CAD build for the part. Positions are in the model's coordinates, mm. Face numbers are marked on the shaded views. A direction names the side the tool comes from. Round coordinates to 2 decimals unless told otherwise and drop trailing zeros. Loops run counter-clockwise (first coordinate to the right, second up) from the corner with the lowest first, then second, coordinate; pieces in that order, holes last. Notation, with made-up numbers: M 59.5,-27.5 L 79.5,-27.5 A15 ccw 79.5,-17.5 Z; hole C 63.25,-11 d1. An arc over 180 degrees is marked long. Use a Markdown table: item, result. Add a question column.
(1) Two-plate mould, pull along Y, no slides. Class the marked faces 1, 2, 3 and 4: released by +Y, released by -Y, zero draft, split by the parting line, or undercut.
(2) Which spindle directions (+Z, -Z, +X, -X, +Y, -Y) get a long thin tool onto all of the face, cutting with end or side? Do the marked faces 5 and 6. Say none if no direction does.
(3) Band-saw the part on A-A, the plane y = 0. Write the cut outline in (x, z), and give its area (3 significant figures).
(4) Wall check: L1, parallel to Y at x = 0, z = 57; L2, parallel to Y at x = 0, z = 48.5; L3, parallel to Z at x = 21, y = 32. Give the ranges that are in metal, low to high.
(5) Band-saw the part on C-C, the plane z = -35.5. Write the cut outline in (x, y), and give its area (3 significant figures).
(6) Flat gauge pins, fed straight in: P1, Ø10, axis at x = 26, z = 6.5, coming from the -Y side; P2, Ø12, axis at y = 32, z = 14.5, coming from the +X side; P3, Ø1.5, axis at x = -9.5, z = -12.5, coming from the +Y side. Where does each tip first touch, or does it go through?
(7) Band-saw the part on D-D, the plane z = -20. Write the cut outline in (x, y).
from build123d import *

# Parameters (mm, degrees)
F2_R     = 19.05
F3_DEPTH = 6.35
F4_R     = 19.05
F5_DEPTH = 16.002


with BuildPart() as f1:
    # F0 (on Front) → F1 (revolve)
    with BuildSketch(Plane.XZ):
        with BuildLine():
            Line((0, -53.330265), (0, 60.969735))
            Line((0, 60.969735), (-40.845792, 60.969735))
            ThreePointArc((-40.845792, 60.969735), (-43.464082, 59.927524), (-44.649926, 57.371076))
            Line((-44.649926, 57.371076), (-50.8, -53.330265))
            Line((-50.8, -53.330265), (0, -53.330265))
        make_face()
    revolve(axis=Axis((0, 0, 3.819735), (0, 0, -1)))

    # F2 (on face) → F3 (join)
    with BuildSketch(Plane(origin=(0, 0, -53.330265), x_dir=(1, 0, 0), z_dir=(0, 0, -1))):
        Circle(F2_R)
    extrude(amount=F3_DEPTH)

    # F4 (on face) → F5 (cut)
    with BuildSketch(Plane.XY.offset(60.969735)):
        Circle(F4_R)
    extrude(amount=-F5_DEPTH, mode=Mode.SUBTRACT)


solid = f1.part
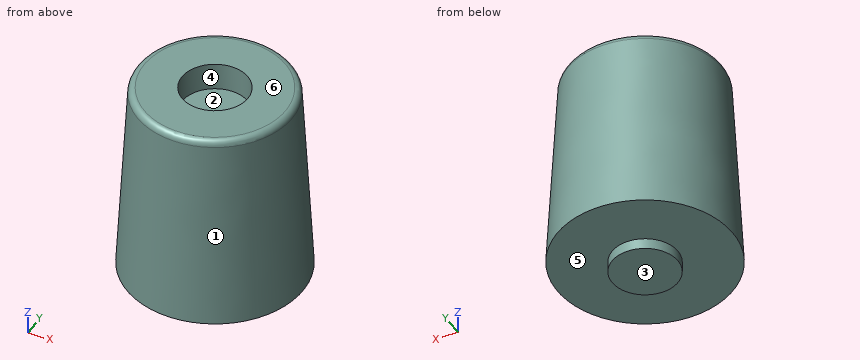
Return value:
| question | item | result |
|---|---|---|
| 1 | face 1 | split by the parting line |
| 1 | face 2 | undercut |
| 1 | face 3 | zero draft |
| 1 | face 4 | undercut |
| 2 | face 5 | -Z |
| 2 | face 6 | +Z, +X, -X, +Y, -Y |
| 3 | outline | M -50.8,-53.33 L -19.05,-53.33 L -19.05,-59.68 L 19.05,-59.68 L 19.05,-53.33 L 50.8,-53.33 L 44.65,57.37 A3.81 ccw 40.85,60.97 L 19.05,60.97 L 19.05,44.97 L -19.05,44.97 L -19.05,60.97 L -40.85,60.97 A3.81 ccw -44.65,57.37 Z |
| 3 | area | 10,500 mm^2 |
| 4 | L1 | -44.67 to -19.05, 19.05 to 44.67 |
| 4 | L2 | -45.14 to -19.05, 19.05 to 45.14 |
| 4 | L3 | -53.33 to 60.97 |
| 5 | outline | C 0,0 d99.62 |
| 5 | area | 7,790 mm^2 |
| 6 | P1 | y = -42.6 |
| 6 | P2 | x = 39.21 |
| 6 | P3 | y = 47.74 |
| 7 | outline | C 0,0 d97.9 |
